```python
from build123d import *

# Parameters (mm, degrees)
BOSS_EXTRUDE1_DEPTH    = 17
SPLIT2_SURFACE_1_BACK  = 26.421
SPLIT2_SURFACE_1_DEPTH = 52.842
SPLIT2_SURFACE_2_BACK  = 26.421
SPLIT2_SURFACE_2_DEPTH = 52.842
SKETCH13_W             = 5.8
SKETCH13_H             = 8.5
BOSS_EXTRUDE10_DEPTH   = 3
FILLET7_R              = 4
SPLIT3_SURFACE_3_BACK  = 34.598
SPLIT3_SURFACE_3_DEPTH = 69.196
SPLIT3_SURFACE_4_BACK  = 34.598
SPLIT3_SURFACE_4_DEPTH = 69.196
CUT_EXTRUDE1_DEPTH     = 1.5
CUT_EXTRUDE2_DEPTH     = 29.664263465
FILLET_1_R             = 1
FILLET_2_R             = 1
FILLET_3_R             = 1.5
CUT_EXTRUDE_START      = 11.5
SKETCH_1_W             = 75.774826167
SKETCH_1_H             = 36.419346407
CUT_EXTRUDE_1_DEPTH    = 10


with BuildPart() as part:
    # Sketch1 → Boss-Extrude1 (new body)
    with BuildSketch(Plane.XY):
        Polygon((0, 0), (1.5, 0), (1.5, 10), (13.5, 10), (13.5, 0), (15, 0), (15, 11.5), (0, 11.5), (0, 10), align=None)
    extrude(amount=BOSS_EXTRUDE1_DEPTH)


with BuildPart() as body_2:
    # Split2: the piece behind the surface
    add(part.part)
    # Split2 surface: a surface, the sketch's curves swept straight by 52.842 mm
    with BuildLine(Plane.XZ.offset(-SPLIT2_SURFACE_1_BACK), mode=Mode.PRIVATE) as split2_surface_1_path:
        Line((15, 8), (0, 8))
    split2_surface_1 = Shell.extrude(split2_surface_1_path.wire(), (0 * SPLIT2_SURFACE_1_DEPTH, -1 * SPLIT2_SURFACE_1_DEPTH, 0 * SPLIT2_SURFACE_1_DEPTH))
    split(bisect_by=split2_surface_1, keep=Keep.BOTTOM)


with BuildPart() as part_1:
    add(part.part)

    # Split2: split by a surface, the side it looks to stays
    # Split2 surface: a surface, the sketch's curves swept straight by 52.842 mm
    with BuildLine(Plane.XZ.offset(-SPLIT2_SURFACE_2_BACK), mode=Mode.PRIVATE) as split2_surface_2_path:
        Line((15, 8), (0, 8))
    split2_surface_2 = Shell.extrude(split2_surface_2_path.wire(), (0 * SPLIT2_SURFACE_2_DEPTH, -1 * SPLIT2_SURFACE_2_DEPTH, 0 * SPLIT2_SURFACE_2_DEPTH))
    split(bisect_by=split2_surface_2, keep=Keep.TOP)


with BuildPart() as body_2_1:
    add(body_2.part)

    # Combine2: union part
    add(part_1.part)

    # Sketch13 → Boss-Extrude10 (add)
    with BuildSketch(Plane.XZ):
        with Locations((-2.9, 4.25)):
            Rectangle(SKETCH13_W, SKETCH13_H)
        with Locations((17.9, 4.25)):
            Rectangle(SKETCH13_W, SKETCH13_H)
    extrude(amount=-BOSS_EXTRUDE10_DEPTH)

    # Fillet7
    fillet7_edges = [body_2_1.edges().sort_by_distance(p)[0] for p in [
        (20.8, 1.5, 8.5),
        (20.8, 1.5, 0),
        (-5.8, 1.5, 0),
        (-5.8, 1.5, 8.5),
    ]]
    fillet(fillet7_edges, radius=FILLET7_R)


with BuildPart() as body_2_2:
    # Split3: the piece behind the surface
    add(body_2_1.part)
    # Split3 surface: a surface, the sketch's curves swept straight by 69.196 mm
    with BuildLine(Plane.ZY.offset(-SPLIT3_SURFACE_3_BACK), mode=Mode.PRIVATE) as split3_surface_3_path:
        Line((0, 3), (17, 3))
    split3_surface_3 = Shell.extrude(split3_surface_3_path.wire(), (-1 * SPLIT3_SURFACE_3_DEPTH, 0 * SPLIT3_SURFACE_3_DEPTH, 0 * SPLIT3_SURFACE_3_DEPTH))
    split(bisect_by=split3_surface_3, keep=Keep.BOTTOM)

    # Sketch16 → Cut-Extrude1 (cut)
    with BuildSketch(Plane(origin=(0, 3, 0), x_dir=(1, 0, 0), z_dir=(0, 1, 0))):
        Polygon((-4, -2.806624327), (-4, -5.693375673), (-1.5, -7.136751346), (1, -5.693375673), (1, -2.806624327), (-1.5, -1.363248654), align=None)
        Polygon((14, -5.693375673), (14, -2.806624327), (16.5, -1.363248654), (19, -2.806624327), (19, -5.693375673), (16.5, -7.136751346), align=None)
    extrude(amount=-CUT_EXTRUDE1_DEPTH, mode=Mode.SUBTRACT)

    # Sketch17 → Cut-Extrude2 (cut, through all)
    with BuildSketch(Plane(origin=(0, 1.5, 0), x_dir=(1, 0, 0), z_dir=(0, 1, 0))):
        with BuildLine():
            Line((16.5, -5.25), (14, -5.25))
            Line((14, -5.25), (14, -3.25))
            Line((14, -3.25), (16.5, -3.25))
            ThreePointArc((16.5, -3.25), (17.5, -4.25), (16.5, -5.25))
        make_face()
        with BuildLine():
            Line((1, -3.25), (1, -5.25))
            Line((1, -5.25), (-1.5, -5.25))
            ThreePointArc((-1.5, -5.25), (-2.5, -4.25), (-1.5, -3.25))
            Line((-1.5, -3.25), (1, -3.25))
        make_face()
    extrude(amount=-CUT_EXTRUDE2_DEPTH, mode=Mode.SUBTRACT)


with BuildPart() as body_2_3:
    add(body_2_1.part)

    # Split3: split by a surface, the side it looks to stays
    # Split3 surface: a surface, the sketch's curves swept straight by 69.196 mm
    with BuildLine(Plane.ZY.offset(-SPLIT3_SURFACE_4_BACK), mode=Mode.PRIVATE) as split3_surface_4_path:
        Line((0, 3), (17, 3))
    split3_surface_4 = Shell.extrude(split3_surface_4_path.wire(), (-1 * SPLIT3_SURFACE_4_DEPTH, 0 * SPLIT3_SURFACE_4_DEPTH, 0 * SPLIT3_SURFACE_4_DEPTH))
    split(bisect_by=split3_surface_4, keep=Keep.TOP)

    # Combine3: union body 2 2
    add(body_2_2.part)

    # Скругление1
    fillet_1_edges = [body_2_3.edges().sort_by_distance(p)[0] for p in [
        (0, 3, 1.114637029),
        (0, 3, 7.385362971),
        (15, 3, 7.385362971),
        (15, 3, 1.114637029),
    ]]
    fillet(fillet_1_edges, radius=FILLET_1_R)

    # Скругление2
    fillet_2_edges = [body_2_3.edges().sort_by_distance(p)[0] for p in [
        (0, 2, 8.5),
        (15, 2, 8.5),
        (0, 11.5, 8.5),
        (15, 11.5, 8.5),
    ]]
    fillet(fillet_2_edges, radius=FILLET_2_R)

    # Скругление3
    fillet_3_edges = [body_2_3.edges().sort_by_distance(p)[0] for p in [
        (13.5, 10, 8.5),
        (1.5, 10, 8.5),
    ]]
    fillet(fillet_3_edges, radius=FILLET_3_R)

    # Эскиз1 → Вырез-Вытянуть1 (cut)
    with BuildSketch(Plane.XY.offset(CUT_EXTRUDE_START)):
        with Locations((-10.82260141, 13.923178903)):
            Rectangle(SKETCH_1_W, SKETCH_1_H)
    extrude(amount=CUT_EXTRUDE_1_DEPTH, mode=Mode.SUBTRACT)


solid = body_2_3.part
```
Read the model definition and answer for the solid it produces. Units are mm, in the model's axes. A direction names the side the tool comes from. Give positions to 0.01 mm unless a question says otherwise; leave off trailing zeros. Write each loop counter-clockwise with the first axis right and the second up, starting at its lowest first coordinate (ties: lowest second). Pieces come first, ordered by that corner, then holes. Notation, with made-up numbers: M -19.75,17 L -7.75,17 A33 cw -7.75,52 Z; hole C -14,-36 d3. An arc over 180 degrees is marked long. Put each result on its own line as item: value. Start each with the question number.
1. Consider line 1 along X through (y, z) = (7.75, 5.5); line 2 along X through (y, z) = (2.5, 5.5); line 3 along Y through (x, z) = (7, 9.75). Determine where each line is inside the solid, lowest interval first.
2. The part is cut by section D-D, the plane x = -0.5. Give the vertices of the cut face in (y, z).
3. Each of these flat-tipped pins is pushed along its axis until it touches: pin 1 Ø1.5 at (x, z) = (-0.5, 4.5) entering from +Y; pin 2 Ø0.6 at (x, y) = (16.5, 2) entering from +Z; pin 3 Ø2.5 at (y, z) = (2.5, 7.5) entering from -X; pin 4 Ø6 at (y, z) = (2.5, 2) entering from +X. Where does it stop, or does it pass through?
4. For a pull along Z with two mould halves and no side action, classify faces 4 (the cylindrical face through (-0.2, 3.4, 7.5)), 5 (the cylindrical face through (19.659, 1.521, 1.203)), 6 (the flat face through (1, 2, 4)), 7 (the cylindrical face through (19.659, 1.521, 7.297)) as released by +Z, released by -Z, zero draft, split by the parting line, or undercut.
5. Which of the six approach directions +Z, -Z, +X, -X, +Y, -Y give full straight-line access (tool end or side, diameter ignored) to faces 1 (the flat face through (-1.4, 1.5, 8.5)), 2 (the flat face through (13.5, 4, 6)), 3 (the cylindrical face through (-2.5, 0.8, 4.3))?
6. The part is cut by section C-C, the plane y = 8. Give the vertices of the cut face in (x, z), and give its area (3 significant figures).
7. The part is cut by section B-B, the plane z = 4.25. Give the vertices of the cut face in (x, y), and give its area (3 significant figures).
8. The part is cut by section A-A, the plane y = 1. Give the vertices of the cut face in (x, z), and give its area (3 significant figures).
Final values:
1. line 1: x = 0 to 1.5, 13.5 to 15
1. line 2: x = -5.67 to -4, 1 to 1.5, 13.5 to 14, 19 to 20.67
1. line 3: y = 10 to 11.5
2. outline: M 0,0 L 3.13,0 L 3.13,1.94 L 1.5,1.94 L 1.5,3.25 L 0,3.25 Z; M 0,5.25 L 1.5,5.25 L 1.5,6.56 L 3.13,6.56 L 3.13,8.63 L 0,8.63 Z
3. pin 1: stops at y = 11.16
3. pin 2: stops at z = 8.5
3. pin 3: stops at x = -5.4
3. pin 4: stops at x = 20.8
4. face 4: zero draft
4. face 5: released by -Z
4. face 6: undercut
4. face 7: released by +Z
5. face 1: +Z, -X, +Y, -Y
5. face 2: +Z, -Z, -Y
5. face 3: +Y, -Y
6. outline: M 0,0 L 1.5,0 L 1.5,11.5 L 0,11.5 Z; M 13.5,0 L 15,0 L 15,11.5 L 13.5,11.5 Z
6. area: 34.5 mm²
7. outline: M -5.8,0 L -2.5,0 L -2.5,1.5 L -4,1.5 L -4,3 L -5.8,3 Z; M 0,3 L 1,3 L 1,0 L 1.5,0 L 1.5,8.5 A1.5 cw 3,10 L 12,10 A1.5 cw 13.5,8.5 L 13.5,0 L 14,0 L 14,3 L 15,3 L 15,10.5 A1 ccw 14,11.5 L 1,11.5 A1 ccw 0,10.5 Z; M 17.5,0 L 20.8,0 L 20.8,3 L 19,3 L 19,1.5 L 17.5,1.5 Z
7. area: 62.3 mm²
8. outline: M -5.8,4 A4 ccw -1.8,0 L 1.5,0 L 1.5,11.5 L 0,11.5 L 0,9.5 A1 cw -1,8.5 L -1.8,8.5 A4 ccw -5.8,4.5 Z; M 13.5,0 L 16.8,0 A4 ccw 20.8,4 L 20.8,4.5 A4 ccw 16.8,8.5 L 16,8.5 A1 cw 15,9.5 L 15,11.5 L 13.5,11.5 Z; hole M -1.5,3.25 L 1,3.25 L 1,5.25 L -1.5,5.25 A1 ccw Z; hole M 14,3.25 L 16.5,3.25 A1 ccw 16.5,5.25 L 14,5.25 Z
8. area: 107 mm²
